Design review of the part built by this model. Coordinates are the model's own, in mm. A direction names the side the tool comes from. Give positions to 0.01 mm unless a question says otherwise; leave off trailing zeros. Loops run counter-clockwise (first coordinate to the right, second up) from the corner with the lowest first, then second, coordinate; pieces in that order, holes last. Notation, with made-up numbers: M 74,59 L 119,59 A33 cw 119,92 Z; hole C -39.75,-12.5 d3. An arc over 180 degrees is marked long. Answer as CSV lines item,"result".
```python
from build123d import *

# Parameters (mm, degrees)
F1_DEPTH = 76.2
F2_R     = 22.225
F3_DEPTH = 254
F4_R     = 12.7
F5_DEPTH = 508


with BuildPart() as f1:
    # F0 (on Front) → F1 (new body)
    with BuildSketch(Plane.XZ):
        with BuildLine():
            ThreePointArc((0, 152.4), (-76.2, 76.2), (0, 0))
            Line((0, 0), (149.225, 0))
            Line((149.225, 0), (149.225, 50.8))
            Line((149.225, 50.8), (73.025, 50.8))
            Line((73.025, 50.8), (73.025, 101.6))
            Line((73.025, 101.6), (149.225, 101.6))
            Line((149.225, 101.6), (149.225, 152.4))
            Line((149.225, 152.4), (0, 152.4))
        make_face()
    extrude(amount=F1_DEPTH)

    # F2 (on face) → F3 (cut)
    with BuildSketch(Plane.XZ.offset(76.2)):
        with Locations((34.925, 80.580235)):
            Circle(F2_R)
    extrude(amount=-F3_DEPTH, mode=Mode.SUBTRACT)

    # F4 (on face) → F5 (cut)
    with BuildSketch(Plane.XY.offset(152.4)):
        with Locations((111.125, -38.1)):
            Circle(F4_R)
    extrude(amount=-F5_DEPTH, mode=Mode.SUBTRACT)


solid = f1.part
```
1. We need section A-A, the plane z = 99. Write out the cut boundary in (x, y) (3 decimals).
Answer block:
outline,"M -72.709,-76.2 L 22.489,-76.2 L 22.489,0 L -72.709,0 Z; M 47.361,-76.2 L 73.025,-76.2 L 73.025,0 L 47.361,0 Z"
2. For P1, Ø1, axis at x = -13.5, y = -51, coming from the -Z side; P2, Ø20.5, axis at x = 111.125, y = -38.1, coming from the -Z side; P3, Ø4, axis at x = -43.5, y = -61, coming from the -Z side, all flat-tipped, find the tip position at first contact; note any pin that passes through.
Answer block:
P1,"z = 1.12"
P2,"through"
P3,"z = 12.29"
3. We need section D-D, the plane y = -65. Write out the cut boundary in (x, z) (3 decimals), plus the area to 3 significant figures.
Answer block:
outline,"M 0,0 L 149.225,0 L 149.225,50.8 L 73.025,50.8 L 73.025,101.6 L 149.225,101.6 L 149.225,152.4 L 0,152.4 A76.2 ccw Z; hole C 34.925,80.58 d44.45"
area,"26,400 mm²"
4. We need section B-B, the plane y = -38.1. Write out the cut boundary in (x, z) (3 decimals).
Answer block:
outline,"M 0,0 L 98.425,0 L 98.425,50.8 L 73.025,50.8 L 73.025,101.6 L 98.425,101.6 L 98.425,152.4 L 0,152.4 A76.2 ccw Z; M 123.825,0 L 149.225,0 L 149.225,50.8 L 123.825,50.8 Z; M 123.825,101.6 L 149.225,101.6 L 149.225,152.4 L 123.825,152.4 Z; hole C 34.925,80.58 d44.45"
5. The part is to be moulded in two halves that separate along Y. For faces 3 (the flat face through (10, 0, 77)), 4 (the cylindrical face through (98.437, -37.542, 127.356)), 5 (the cylindrical face through (98.437, -37.542, 25.756)), 6 (the cylindrical face through (18.544, -38.633, 95.601)), say which applies: pulls with the +Y half, pulls with the -Y half, needs draft (parallel to the pull), parting line crosses it, or undercut.
Answer block:
face 3,"pulls with the +Y half"
face 4,"undercut"
face 5,"undercut"
face 6,"needs draft"
6. We need section C-C, the plane x = 104.5. Write out the cut boundary in (y, z).
Answer block:
outline,"M -76.2,0 L -48.94,0 L -48.94,50.8 L -76.2,50.8 Z; M -76.2,101.6 L -48.94,101.6 L -48.94,152.4 L -76.2,152.4 Z; M -27.26,0 L 0,0 L 0,50.8 L -27.26,50.8 Z; M -27.26,101.6 L 0,101.6 L 0,152.4 L -27.26,152.4 Z"
7. For faces 1 (the flat face through (112, -21, 50.8)), 2 (the flat face through (149.225, -38, 25)), list the 3-axis set-ups (+Z, -Z, +X, -X, +Y, -Y) from which the entire face can be reached by the end or side of a thin tool; tool diameter is ignored.
Answer block:
face 1,"+X, +Y, -Y"
face 2,"+Z, -Z, +X, +Y, -Y"
8. To check wall thickness, follow L1, parallel to Z at x = 105.5, y = -26; L2, parallel to X at y = -47.5, z = 87 (3 decimals); L3, parallel to Z at x = 54, y = -56. State the ranges of each line that lie inside material, in increasing order. Write a range as [from, to].
Answer block:
L1,"[0, 50.8], [101.6, 152.4]"
L2,"[-75.431, 13.647], [56.203, 73.025]"
L3,"[0, 69.17], [91.99, 152.4]"
